Design review of the part built by this model. Coordinates are the model's own, in mm. A direction names the side the tool comes from. Give positions to 0.01 mm unless a question says otherwise; leave off trailing zeros. Loops run counter-clockwise (first coordinate to the right, second up) from the corner with the lowest first, then second, coordinate; pieces in that order, holes last.
from build123d import *

# Parameters (mm, degrees)
F0_R      = 304.8
F1_DEPTH  = 25.4
F3_R      = 304.8
F4_DEPTH  = 25.4
F7_W      = 139.7
F7_H      = 38.1
F7_W_2    = 38.1
F7_H_2    = 139.7
F8_DEPTH  = 431.8
F9_W      = 139.7
F9_H      = 38.1
F9_W_2    = 38.1
F9_H_2    = 139.7
F10_DEPTH = 457.2
F6_R      = 304.8
F11_DEPTH = 50.8


with BuildPart() as f1:
    # F0 (on Top) → F1 (new body)
    with BuildSketch(Plane.XY):
        Circle(F0_R)
    extrude(amount=F1_DEPTH)



with BuildPart() as f4:
    # F3 (on offset) → F4 (new body)
    with BuildSketch(Plane.XY.offset(457.2)):
        Circle(F3_R)
    extrude(amount=F4_DEPTH)


with BuildPart() as f1_1:
    add(f1.part)

    add(f4.part)  # F8 merges F4
    # F7 (on face) → F8 (join, through all)
    with BuildSketch(Plane.XY.offset(25.4)):
        with Locations((-234.95, 19.05)):
            Rectangle(F7_W, F7_H)
        Polygon((152.4, 263.9645430735), (82.55, 142.9807941648), (114.2904353584, 121.9058146094), (184.1404353584, 242.8895635181), align=None)
        Polygon((152.4, -263.9645430735), (82.55, -142.9807941648), (49.5544321158, -162.0307941648), (118.2091195432, -280.9442009667), align=None)
        Rectangle(F7_W_2, F7_H_2)
    extrude(amount=F8_DEPTH)

    # F9 (on face) → F10 (join, through all)
    with BuildSketch(Plane.XY.offset(914.4)):
        with Locations((-234.95, 19.05)):
            Rectangle(F9_W, F9_H)
        Polygon((152.4, 263.9645430735), (82.55, 142.9807941648), (114.2904353584, 121.9058146094), (184.1404353584, 242.8895635181), align=None)
        Polygon((152.4, -263.9645430735), (82.55, -142.9807941648), (49.5544321158, -162.0307941648), (118.2091195432, -280.9442009667), align=None)
        Rectangle(F9_W_2, F9_H_2)
    extrude(amount=-F10_DEPTH)

    # F6 (on offset) → F11 (join)
    with BuildSketch(Plane.XY.offset(914.4)):
        Circle(F6_R)
    extrude(amount=F11_DEPTH)


solid = f1_1.part
Q1. Take a section at A-A (z = 693.5). Give the boundary of the cut face in (x, y).
Results:
outline: (-304.8, 0) - (-165.1, 0) - (-165.1, 38.1) - (-304.8, 38.1) - close; (-19.05, -69.85) - (19.05, -69.85) - (19.05, 69.85) - (-19.05, 69.85) - close; (49.55, -162.03) - (118.21, -280.94) - (152.4, -263.96) - (82.55, -142.98) - close; (82.55, 142.98) - (114.29, 121.91) - (184.14, 242.89) - (152.4, 263.96) - close
Q2. Insertion check: pin 1 (1 mm diameter, centred on x = -31.5, y = -105, fed in from -Z); pin 2 (19 mm diameter, centred on x = -7, z = 717.5, fed in from +Y); pin 3 (4 mm diameter, centred on x = 170, z = 452, fed in from -Y); pin 4 (1.5 mm diameter, centred on y = 138.5, z = 694, fed in from +X). Each pin has a flat end and moves straight along its axis. Give the tip position at first contact, or say it passes through.
Results:
pin 1: stops at z = 0
pin 2: stops at y = 69.85
pin 3: stops at y = 214.93
pin 4: stops at x = 124.3
Q3. Tool access review of faces 1 (the face through (63, 4, 482.6)), 2 (the face through (66.283, -152.372, 701.523)), 3 (the face through (148.726, 181.551, 238.277)), 4 (the face through (83.401, -220.655, 701.523)): name each direction out of +Z, -Z, +X, -X, +Y, -Y from which nothing blocks a thin tool from reaching the whole face with its end or side.
Results:
face 1: none
face 2: -X, +Y
face 3: +X
face 4: -X, -Y
Q4. Take a section at D-D (x = 93.5). Give the boundary of the cut face in (y, z).
Results:
outline: (-290.1, 0) - (290.1, 0) - (290.1, 25.4) - (161.95, 25.4) - (161.95, 457.2) - (290.1, 457.2) - (290.1, 482.6) - (161.95, 482.6) - (161.95, 914.4) - (290.1, 914.4) - (290.1, 965.2) - (-290.1, 965.2) - (-290.1, 914.4) - (-238.15, 914.4) - (-238.15, 482.6) - (-290.1, 482.6) - (-290.1, 457.2) - (-238.15, 457.2) - (-238.15, 25.4) - (-290.1, 25.4) - close; hole (-161.95, 25.4) - (135.71, 25.4) - (135.71, 457.2) - (-161.95, 457.2) - close; hole (-161.95, 482.6) - (135.71, 482.6) - (135.71, 914.4) - (-161.95, 914.4) - close
Q5. Take a section at B-B (x = 0). Give the boundary of the cut face in (y, z), plus the area to 3 significant figures.
Results:
outline: (-304.8, 0) - (304.8, 0) - (304.8, 25.4) - (69.85, 25.4) - (69.85, 457.2) - (304.8, 457.2) - (304.8, 482.6) - (69.85, 482.6) - (69.85, 914.4) - (304.8, 914.4) - (304.8, 965.2) - (-304.8, 965.2) - (-304.8, 914.4) - (-69.85, 914.4) - (-69.85, 482.6) - (-304.8, 482.6) - (-304.8, 457.2) - (-69.85, 457.2) - (-69.85, 25.4) - (-304.8, 25.4) - close
area: 183,000 mm2
Q6. Draft analysis for pull direction X (two halves, no side actions). For faces 5 (the face through (-165.1, 19, 702)), 6 (the face through (-241.879, -185.466, 939.444)), 7 (the face through (83.401, -220.655, 238.277)), 8 (the face through (168.49, 253.28, 238.28)), state which applies: pulls with the +X half, pulls with the -X half, needs draft (parallel to the pull), parting line crosses it, or undercut.
Results:
face 5: undercut
face 6: parting line crosses it
face 7: pulls with the -X half
face 8: pulls with the +X half
Q7. Take a section at C-C (x = 237). Give the boundary of the cut face in (y, z), plus the area to 3 significant figures.
Results:
outline: (-191.66, 0) - (191.66, 0) - (191.66, 25.4) - (-191.66, 25.4) - close; (-191.66, 457.2) - (191.66, 457.2) - (191.66, 482.6) - (-191.66, 482.6) - close; (-191.66, 914.4) - (191.66, 914.4) - (191.66, 965.2) - (-191.66, 965.2) - close
area: 38,900 mm2
Q8. Wall thickness on line 1 (Z direction, x = 117.5, y = 27.5); line 2 (X direction, y = 31, z = 516); line 3 (X direction, y = 49.5, z = 410.5): over which ranges is each line inside the solid? List them lowest first.
Results:
line 1: z = 0 to 25.4, 457.2 to 482.6, 914.4 to 965.2
line 2: x = -304.8 to -165.1, -19.05 to 19.05
line 3: x = -19.05 to 19.05
